```python
from build123d import *

# Parameters (mm, degrees)
F1_DEPTH        = 16
F2_T            = -2
F3_R            = 4.5
F4_DEPTH        = 9
F6_R            = 2.4
F7_DEPTH        = 5
F3_W            = 2
F3_H            = 112
F8_DEPTH        = 16
F9_R            = 1.4
F9_W            = 14
F9_H            = 12
F9_H_2          = 2
F9_R_2          = 1.5
F9_W_2          = 21
F11_DEPTH       = 4
F10_R           = 1.5
F10_W           = 21
F10_H           = 2
F12_DEPTH       = 4
F13_D           = 4
F13_CSINK_D     = 7
F13_CSINK_ANGLE = 60
F14_D           = 7
F14_DEPTH       = 2.001


with BuildPart() as f1:
    # F0 (on Top) → F1 (new body)
    with BuildSketch(Plane.XY):
        with BuildLine():
            Line((-36, -67), (36, -67))
            ThreePointArc((36, -67), (39.5355339059, -65.5355339059), (41, -62))
            Line((41, -62), (41, 62))
            ThreePointArc((41, 62), (39.5355339059, 65.5355339059), (36, 67))
            Line((36, 67), (-36, 67))
            ThreePointArc((-36, 67), (-39.5355339059, 65.5355339059), (-41, 62))
            Line((-41, 62), (-41, -62))
            ThreePointArc((-41, -62), (-39.5355339059, -65.5355339059), (-36, -67))
        make_face()
    extrude(amount=F1_DEPTH)

    # F2
    f2_openings = [f1.faces().sort_by_distance(p)[0] for p in [
        (0, 0, 16),
    ]]
    offset(amount=F2_T, openings=f2_openings)

    # F3 (on face) → F4 (join)
    with BuildSketch(Plane.XY.offset(2)):
        with Locations((-23, 30)):
            Circle(F3_R)
        with Locations((-23, -30)):
            Circle(F3_R)
        with Locations((29, -30)):
            Circle(F3_R)
        with Locations((29, 30)):
            Circle(F3_R)
    extrude(amount=F4_DEPTH)

    # F6 (on mid) → F7 (join)
    with BuildSketch(Plane.XY.offset(11)):
        with Locations((-23, 30)):
            Circle(F6_R)
        with Locations((29, 30)):
            Circle(F6_R)
        with Locations((-23, -30)):
            Circle(F6_R)
        with Locations((29, -30)):
            Circle(F6_R)
    extrude(amount=F7_DEPTH)

    # F3 (on face) → F8 (join)
    with BuildSketch(Plane.XY.offset(2)):
        with BuildLine():
            Line((-37, 56), (-30, 56))
            Line((-30, 56), (-30, 65))
            Line((-30, 65), (-36, 65))
            ThreePointArc((-36, 65), (-38.1213203436, 64.1213203436), (-39, 62))
            Line((-39, 62), (-39, 56))
            Line((-39, 56), (-37, 56))
        make_face()
        with BuildLine():
            Line((36, 65), (30, 65))
            Line((30, 65), (30, 56))
            Line((30, 56), (37, 56))
            Line((37, 56), (39, 56))
            Line((39, 56), (39, 62))
            ThreePointArc((39, 62), (38.1213203436, 64.1213203436), (36, 65))
        make_face()
        with BuildLine():
            Line((30, -56), (30, -65))
            Line((30, -65), (36, -65))
            ThreePointArc((36, -65), (38.1213203436, -64.1213203436), (39, -62))
            Line((39, -62), (39, -56))
            Line((39, -56), (37, -56))
            Line((37, -56), (30, -56))
        make_face()
        with BuildLine():
            Line((-30, -56), (-37, -56))
            Line((-37, -56), (-39, -56))
            Line((-39, -56), (-39, -62))
            ThreePointArc((-39, -62), (-38.1213203436, -64.1213203436), (-36, -65))
            Line((-36, -65), (-30, -65))
            Line((-30, -65), (-30, -56))
        make_face()
        with Locations((-38, 0)):
            Rectangle(F3_W, F3_H)
        with Locations((38, 0)):
            Rectangle(F3_W, F3_H)
    extrude(amount=F8_DEPTH)

    # F9 (on face) → F11 (cut)
    with BuildSketch(Plane(origin=(-41, 0, 0), x_dir=(0, -1, 0), z_dir=(-1, 0, 0))):
        with Locations((-13, 10)):
            Circle(F9_R)
        with Locations((13, 10)):
            Circle(F9_R)
        with Locations((0, 10)):
            Rectangle(F9_W, F9_H)
        with Locations((0, 17)):
            Rectangle(F9_W, F9_H_2)
        with Locations((23.825, 10)):
            Circle(F9_R_2)
        with Locations((49.825, 10)):
            Circle(F9_R_2)
        with Locations((36.825, 17)):
            Rectangle(F9_W_2, F9_H_2)
        Polygon((47.325, 16), (26.325, 16), (28.825, 4), (44.825, 4), align=None)
    extrude(amount=-F11_DEPTH, mode=Mode.SUBTRACT)

    # F10 (on face) → F12 (cut)
    with BuildSketch(Plane.YZ.offset(41)):
        with Locations((-13, 10)):
            Circle(F10_R)
        with Locations((13, 10)):
            Circle(F10_R)
        with Locations((0, 17)):
            Rectangle(F10_W, F10_H)
        Polygon((10.5, 16), (-10.5, 16), (-8, 4), (8, 4), align=None)
    extrude(amount=-F12_DEPTH, mode=Mode.SUBTRACT)

    # F13 (through all)
    with Locations(Plane(origin=(0, 0, 2), x_dir=(1, 0, 0), z_dir=(0, 0, -1))):
        with Locations((34.5, -60.5), (-34.5, -60.5), (-34.5, 60.5), (34.5, 60.5)):
            CounterSinkHole(F13_D / 2, F13_CSINK_D / 2, counter_sink_angle=F13_CSINK_ANGLE)

    # F14 (through all, one way)
    with BuildSketch(Plane.XY.offset(2)):
        with Locations((-34.5, 60.5), (-34.5, -60.5), (34.5, 60.5), (34.5, -60.5)):
            Circle(F14_D / 2)
    extrude(amount=-F14_DEPTH, mode=Mode.SUBTRACT)


solid = f1.part
```
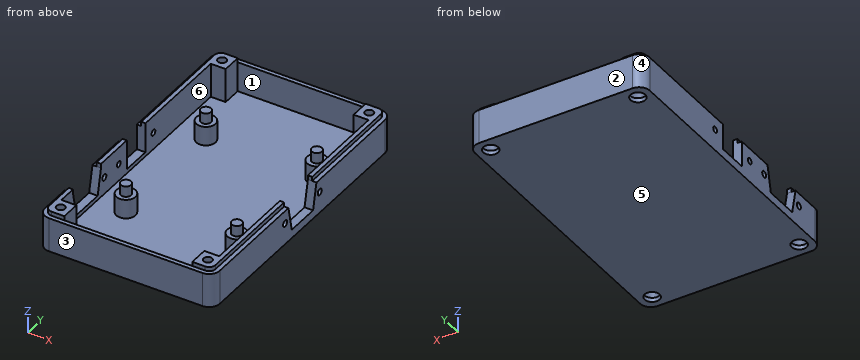
Build history of the part. All positions in model axes, mm. Face numbers are marked on the shaded views. A direction names the side the tool comes from. Round coordinates to 2 decimals unless told otherwise and drop trailing zeros. Order: outer loops, then holes, each group sorted by start corner. A loop starts at its lowest first (then second) coordinate and runs counter-clockwise, first axis right, second up. Notation, with made-up numbers: (75.25, 44) - (98.25, 44) arc R23 ccw to (98.25, 82) - close; hole circle Ø6 at (82, 58.25). An arc over 180 degrees is marked (long way). Use a Markdown table: item, result.
1) Flat gauge pins, fed straight in: pin 1 Ø8 at (x, y) = (-2.5, 42.5) entering from +Z; pin 2 Ø2 at (y, z) = (-24, 17.5) entering from +X; pin 3 Ø1.6 at (y, z) = (45, 17) entering from -X; pin 4 Ø2.5 at (y, z) = (13, 10) entering from +X. Where does each tip first touch, or does it go through?
Recorded:
| item | result |
|---|---|
| pin 1 | stops at z = 2 |
| pin 2 | stops at x = 39 |
| pin 3 | stops at x = -39 |
| pin 4 | passes through |
2) Saw through at D-D on y = -40. Write the cut outline in (x, z).
Recorded:
| item | result |
|---|---|
| outline | (-41, 0) - (41, 0) - (41, 16) - (39, 16) - (39, 18) - (37, 18) - (37, 2) - (-37, 2) - (-37, 4) - (-41, 4) - close |
3) Saw through at B-B on x = -23. Write the cut outline in (y, z).
Recorded:
| item | result |
|---|---|
| outline | (-67, 0) - (67, 0) - (67, 16) - (65, 16) - (65, 2) - (34.5, 2) - (34.5, 11) - (32.4, 11) - (32.4, 16) - (27.6, 16) - (27.6, 11) - (25.5, 11) - (25.5, 2) - (-25.5, 2) - (-25.5, 11) - (-27.6, 11) - (-27.6, 16) - (-32.4, 16) - (-32.4, 11) - (-34.5, 11) - (-34.5, 2) - (-65, 2) - (-65, 16) - (-67, 16) - close |
4) Tool access for the marked faces 1 and 2: list every direction of +Z, -Z, +X, -X, +Y, -Y with a clear straight run to the whole face (end or side of a thin tool).
Recorded:
| item | result |
|---|---|
| face 1 | +Z |
| face 2 | +Z, -Z, +X, -X, +Y |
5) Saw through at A-A on y = 13. Write the cut outline in (x, z), and give its area (3 significant figures).
Recorded:
| item | result |
|---|---|
| outline | (-41, 0) - (41, 0) - (41, 8.5) - (37, 8.5) - (37, 2) - (-37, 2) - (-37, 8.6) - (-41, 8.6) - close; (-41, 11.4) - (-37, 11.4) - (-37, 18) - (-39, 18) - (-39, 16) - (-41, 16) - close; (37, 11.5) - (41, 11.5) - (41, 16) - (39, 16) - (39, 18) - (37, 18) - close |
| area | 261 mm² |
6) Wall check: L1, parallel to X at y = -60.5, z = 10.5; L2, parallel to Y at x = -34.5, z = 0.4; L3, parallel to X at y = 60.5, z = 1.15. Give the ranges that are in metal, low to high.
Recorded:
| item | result |
|---|---|
| L1 | x = -41 to -36.5, -32.5 to -30, 30 to 32.5, 36.5 to 41 |
| L2 | y = -67 to -64, -57 to 57, 64 to 67 |
| L3 | x = -41 to -38, -31 to 31, 38 to 41 |
7) Saw through at C-C on x = -34.5. Write the cut outline in (y, z).
Recorded:
| item | result |
|---|---|
| outline | (-67, 0) - (-64, 0) - (-64, 2) - (-62.5, 4.6) - (-62.5, 18) - (-65, 18) - (-65, 16) - (-67, 16) - close; (-58.5, 4.6) - (-57, 2) - (-57, 0) - (57, 0) - (57, 2) - (58.5, 4.6) - (58.5, 18) - (56, 18) - (56, 2) - (-56, 2) - (-56, 18) - (-58.5, 18) - close; (62.5, 4.6) - (64, 2) - (64, 0) - (67, 0) - (67, 16) - (65, 16) - (65, 18) - (62.5, 18) - close |
8) Pull direction Y, two halves, no side cores. Call the marked faces 3, 4, 5 and 6: pulls with the +Y half, pulls with the -Y half, needs draft (parallel to the pull), parting line crosses it, or undercut.
Recorded:
| item | result |
|---|---|
| face 3 | pulls with the -Y half |
| face 4 | pulls with the +Y half |
| face 5 | needs draft |
| face 6 | undercut |
